Autodesk Inventor part; units mm, degrees
ref_plane "YZ Plane" through (0, 0, 0) normal (1, 0, 0) x (0, 1, 0)
ref_plane "XZ Plane" through (0, 0, 0) normal (0, 1, 0) x (-1, 0, 0)
ref_plane "XY Plane" through (0, 0, 0) normal (0, 0, 1) x (1, 0, 0)
sketch "Sketch1" plane through (0, 0, 0) normal (0, 0, 1) x (1, 0, 0)
  circle A0 centre (0, 0) radius 11
  dimension "d0" = 22
extrude "Extrusion1" add sketch "Sketch1" along normal blind 10
sketch "Sketch2" plane through (0, 0, 10) normal (0, 0, 1) x (1, 0, 0)
  circle A0 centre (0, 0) radius 11
  circle A1 centre (0, 0) radius 8
  circle A2 centre (-8, 0) radius 1
  circle A3 centre (0, 8) radius 1
  circle A4 centre (8, 0) radius 1
  circle A5 centre (0, -8) radius 1
  dimension "d3" = 16
  dimension "d4" = 2
  dimension "d5" = 2
  dimension "d6" = 2
  dimension "d7" = 2
extrude "Extrusion2" cut sketch "Sketch2" against normal blind 10 contours A1 A4 | A1 A4 | A3 A1 | A1 A3 | A5 A1 | A1 A5 | A2 A1 | A1 A2
sketch "Sketch3" plane through (0, 0, 10) normal (0, 0, 1) x (1, 0, 0)
  circle A0 centre (8, 0) radius 1
  circle A1 centre (0, -8) radius 1
  circle A2 centre (-8, 0) radius 1
  circle A3 centre (0, 8) radius 1
  circle A4 centre (0, 0) radius 11
extrude "Extrusion3" cut sketch "Sketch3" against normal blind 9.525
sketch "Sketch4" plane through (0, 0, 0.475) normal (0, 0, 1) x (1, 0, 0)
  circle A0 centre (0, 8) radius 1
  circle A1 centre (-8, 0) radius 1
  circle A2 centre (0, -8) radius 1
  circle A3 centre (8, 0) radius 1
  circle A4 centre (0, 0) radius 11
extrude "Extrusion4" add sketch "Sketch4" against normal blind 9.525
properties part number "Spacer"
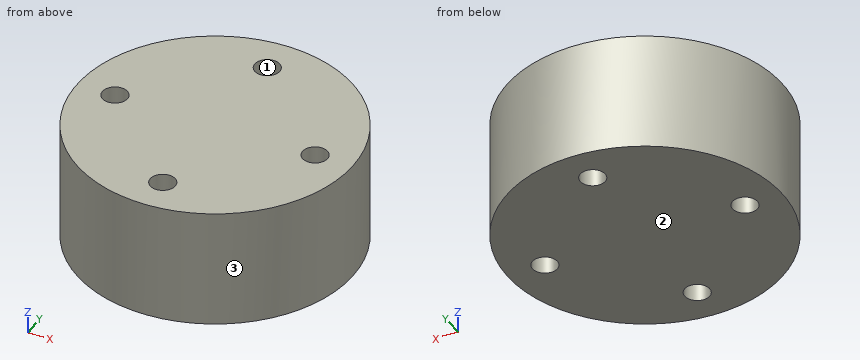
Geometry: final body of the model. Coordinates: model frame, mm. Face numbers are marked on the shaded views. Round coordinates to 2 decimals unless told otherwise and drop trailing zeros. Order: outer loops, then holes, each group sorted by start corner. A loop starts at its lowest first (then second) coordinate and runs counter-clockwise, first axis right, second up.
Q1. Material intervals for probe 1 along Y at (x, z) = (0, -6.25); probe 2 along Y at (x, z) = (-0.5, -4.75); probe 3 along Y at (x, z) = (8, -7), sorted ascending.
Result sheet:
probe 1: y = -11 to -9, -7 to 7, 9 to 11
probe 2: y = -10.99 to -8.87, -7.13 to 7.13, 8.87 to 10.99
probe 3: y = -7.55 to -1, 1 to 7.55
Q2. Mould query, pull axis Y, two halves, no side actions, for the marked faces 1, 2 and 3. Classes: released by +Y, released by -Y, zero draft, split by the parting line, or undercut.
Result sheet:
face 1: undercut
face 2: zero draft
face 3: split by the parting line
Q3. Section C-C, the plane y = 7.5. Output: boundary loops of the cut face in (x, z) (3 decimals).
Result sheet:
outline: (-8.047, -9.05) - (-0.866, -9.05) - (-0.866, 0.475) - (-8.047, 0.475) - close; (0.866, -9.05) - (8.047, -9.05) - (8.047, 0.475) - (0.866, 0.475) - close
Q4. Section D-D, the plane x = -8. Output: boundary loops of the cut face in (y, z) (3 decimals).
Result sheet:
outline: (-7.55, -9.05) - (-1, -9.05) - (-1, 0.475) - (-7.55, 0.475) - close; (1, -9.05) - (7.55, -9.05) - (7.55, 0.475) - (1, 0.475) - close
Q5. Pin query (flat end, axial travel): pin 1 (3 mm diameter, centred on x = 5, z = -3, fed in from -Y); pin 2 (1.8 mm diameter, centred on x = -8, y = 0, fed in from +Z); pin 3 (2 mm diameter, centred on x = 8, z = -2.5, fed in from -Y); pin 4 (2 mm diameter, centred on y = 2, z = -0.5, fed in from -X). Return the tip coordinate at first contact, or that it passes through.
Result sheet:
pin 1: stops at y = -10.43
pin 2: passes through
pin 3: stops at y = -8.49
pin 4: stops at x = -10.95
Q6. Section A-A, the plane x = 0. Output: boundary loops of the cut face in (y, z) (3 decimals), and give its area (3 significant figures).
Result sheet:
outline: (-11, -9.05) - (-9, -9.05) - (-9, 0.475) - (-11, 0.475) - close; (-7, -9.05) - (7, -9.05) - (7, 0.475) - (-7, 0.475) - close; (9, -9.05) - (11, -9.05) - (11, 0.475) - (9, 0.475) - close
area: 171 mm2
Q7. Section B-B, the plane z = -5. Output: boundary loops of the cut face in (x, y).
Result sheet:
outline: circle Ø22 at (0, 0); hole circle Ø2 at (-8, 0); hole circle Ø2 at (0, -8); hole circle Ø2 at (0, 8); hole circle Ø2 at (8, 0)
